CAD build for the part. Positions are in the model's coordinates, mm. A direction names the side the tool comes from. Round coordinates to 2 decimals unless told otherwise and drop trailing zeros. Loops run counter-clockwise (first coordinate to the right, second up) from the corner with the lowest first, then second, coordinate; pieces in that order, holes last. Notation, with made-up numbers: (11.25, -35.5) - (52.25, -35.5) arc R16 cw to (52.25, -8.5) - close; hole circle Ø1 at (-38, -35). An arc over 180 degrees is marked (long way). Use one line per item in the form item = value.
from build123d import *

# Parameters (mm, degrees)
CROQUIS1_R              = 1.475
SALIENTE_EXTRUIR1_DEPTH = 7.8
CROQUIS2_R              = 2.7
SALIENTE_EXTRUIR2_DEPTH = 3
CORTAR_EXTRUIR1_DEPTH   = 2.5
REDONDEO1_R             = 0.3


with BuildPart() as part:
    # Croquis1 → Saliente-Extruir1 (new body)
    with BuildSketch(Plane.XY):
        Circle(CROQUIS1_R)
    extrude(amount=SALIENTE_EXTRUIR1_DEPTH)

    # Croquis2 → Saliente-Extruir2 (add)
    with BuildSketch(Plane(origin=(0, 0, 0), x_dir=(-1, 0, 0), z_dir=(0, 0, -1))):
        Circle(CROQUIS2_R)
    extrude(amount=SALIENTE_EXTRUIR2_DEPTH)

    # Croquis3 → Cortar-Extruir1 (cut)
    with BuildSketch(Plane(origin=(0, 0, -3), x_dir=(-1, 0, 0), z_dir=(0, 0, -1))):
        Polygon((0, -1.776735144), (1.53869777, -0.888367572), (1.53869777, 0.888367572), (0, 1.776735144), (-1.53869777, 0.888367572), (-1.53869777, -0.888367572), align=None)
    extrude(amount=-CORTAR_EXTRUIR1_DEPTH, mode=Mode.SUBTRACT)

    # Redondeo1
    redondeo1_edges = [part.edges().sort_by_distance(p)[0] for p in [
        (2.7, 0, -3),
    ]]
    fillet(redondeo1_edges, radius=REDONDEO1_R)


solid = part.part
1) Tool access for faces 1 (the cylindrical face through (0.585, -2.636, -1.331)), 2 (the flat face through (-1.2, -1.2, 0)), 3 (the flat face through (-0.78, 1.326, -1.768)): list every direction of +Z, -Z, +X, -X, +Y, -Y with a clear straight run to the whole face (end or side of a thin tool).
Report:
face_1 = +Z, -Z
face_2 = +Z
face_3 = -Z
2) Drill centre lines: probe 1 along Z at (x, y) = (0.3, 2.4); probe 2 along Z at (x, y) = (1.1, 0.6); probe 3 along Y at (x, z) = (1.25, 5). Where is each one in solid material? Low to high.
Report:
probe_1 = -3 to 0
probe_2 = -0.5 to 7.8
probe_3 = -0.78 to 0.78
3) Flat gauge pins, fed straight in: pin 1 (3 mm diameter, centred on y = 1, z = 0, fed in from +X); pin 2 (3 mm diameter, centred on y = 2, z = -1.5, fed in from -X); pin 3 (3 mm diameter, centred on y = -1, z = 4.5, fed in from -X) (3 decimals). Where does each tip first touch, or does it go through?
Report:
pin_1 = 2.7
pin_2 = -2.65
pin_3 = -1.475
4) Slice it at A-A (z = -1.5). Write the cut outline in (x, y), plus the area to 3 significant figures.
Report:
outline = circle Ø5.4 at (0, 0); hole (-1.54, -0.89) - (0, -1.78) - (1.54, -0.89) - (1.54, 0.89) - (0, 1.78) - (-1.54, 0.89) - close
area = 14.7 mm^2
5) Slice it at C-C (z = 5.75). Write the cut outline in (x, y) (3 decimals).
Report:
outline = circle Ø2.95 at (0, 0)
6) Slice it at B-B (y = 0). Write the cut outline in (x, z) (3 decimals).
Report:
outline = (-2.7, -2.7) arc R0.3 ccw to (-2.4, -3) - (-1.539, -3) - (-1.539, -0.5) - (1.539, -0.5) - (1.539, -3) - (2.4, -3) arc R0.3 ccw to (2.7, -2.7) - (2.7, 0) - (1.475, 0) - (1.475, 7.8) - (-1.475, 7.8) - (-1.475, 0) - (-2.7, 0) - close
7) Two-plate mould, pull along X, no slides. Class faces 4 (the cylindrical face through (-1.474, 0.065, 3.845)), 5 (the flat face through (0.76, 1.34, -1.77)), 6 (the flat face through (-2, 0, -3)): +X half, -X half, draft (parallel to the pull), parting line (faces both ways), or undercut.
Report:
face_4 = parting line
face_5 = undercut
face_6 = draft
